Verification items for the finished model (mm, model axes). A direction names the side the tool comes from. Round coordinates to 2 decimals unless told otherwise and drop trailing zeros. Write each loop counter-clockwise with the first axis right and the second up, starting at its lowest first coordinate (ties: lowest second). Pieces come first, ordered by that corner, then holes. Notation, with made-up numbers: (45.5, 64) - (84.5, 64) arc R22 cw to (84.5, 89) - close; hole circle Ø11 at (25.5, -6.75). An arc over 180 degrees is marked (long way). Write each question's results on one line, items separated by ' | '.
```python
from build123d import *

# Parameters (mm, degrees)
SKETCH_1_W          = 96
SKETCH_1_H          = 45
SKETCH_1_R          = 1.75
EXTRUDE_1_DEPTH     = 4
SKETCH_2_W          = 4
SKETCH_2_H          = 45
EXTRUDE_2_DEPTH     = 85
SKETCH_3_W          = 49
SKETCH_3_H          = 45
EXTRUDE_3_DEPTH     = 4
SKETCH_4_W          = 41
SKETCH_4_H          = 4
EXTRUDE_4_DEPTH     = 45
FILLET_1_R          = 4
SKETCH_5_R          = 4.5
CUT_EXTRUDE_1_DEPTH = 4
FILLET_2_R          = 2


with BuildPart() as part:
    # 草图1 → 凸台-拉伸1 (new body)
    with BuildSketch(Plane.XY):
        Rectangle(SKETCH_1_W, SKETCH_1_H)
        with Locations((8.5, 0)):
            Circle(SKETCH_1_R, mode=Mode.SUBTRACT)
        with Locations((-36.5, 0)):
            Circle(SKETCH_1_R, mode=Mode.SUBTRACT)
    extrude(amount=EXTRUDE_1_DEPTH)

    # 草图2 → 凸台-拉伸2 (add)
    with BuildSketch(Plane(origin=(0, 0, 0), x_dir=(-1, 0, 0), z_dir=(0, 0, -1))):
        with Locations((-31, 0)):
            Rectangle(SKETCH_2_W, SKETCH_2_H)
        with Locations((14, 0)):
            Rectangle(SKETCH_2_W, SKETCH_2_H)
    extrude(amount=EXTRUDE_2_DEPTH)

    # 草图3 → 凸台-拉伸3 (add)
    with BuildSketch(Plane(origin=(0, 0, -85), x_dir=(-1, 0, 0), z_dir=(0, 0, -1))):
        with Locations((-8.5, 0)):
            Rectangle(SKETCH_3_W, SKETCH_3_H)
    extrude(amount=EXTRUDE_3_DEPTH)

    # 草图4 → 凸台-拉伸4 (add)
    with BuildSketch(Plane.XZ.offset(22.5)):
        with Locations((8.5, -42)):
            Rectangle(SKETCH_4_W, SKETCH_4_H)
    extrude(amount=-EXTRUDE_4_DEPTH)

    # 圆角1
    fillet_1_edges = [part.edges().sort_by_distance(p)[0] for p in [
        (-16, 0, 0),
        (33, 0, 0),
        (33, 0, -89),
        (-16, 0, -89),
    ]]
    fillet(fillet_1_edges, radius=FILLET_1_R)

    # 草图5 → 切除-拉伸1 (cut)
    with BuildSketch(Plane(origin=(0, 0, -89), x_dir=(-1, 0, 0), z_dir=(0, 0, -1))):
        with Locations((-8.5, 0)):
            Circle(SKETCH_5_R)
    extrude(amount=-CUT_EXTRUDE_1_DEPTH, mode=Mode.SUBTRACT)

    # 圆角2
    fillet_2_edges = [part.edges().sort_by_distance(p)[0] for p in [
        (-48, 0, 4),
        (-48, 0, 0),
        (48, 0, 4),
        (48, 0, 0),
    ]]
    fillet(fillet_2_edges, radius=FILLET_2_R - 0.0001)  # a hair under: the kernel refuses the full size


solid = part.part
```
(1) Go/stop test with flat-tipped pins: pin 1 Ø13.5 at (y, z) = (-9.5, -41.5) entering from -X; pin 2 Ø4 at (x, y) = (37, 2) entering from -Z; pin 3 Ø2 at (x, y) = (8.5, 0) entering from -Z. Record where each tip stops, or that it passes through.
Answer:
pin 1: x = -16 | pin 2: z = -0.54 | pin 3: z = -44
(2) Mould release check, pull along X, two halves, no side actions. Record for faces 5 (the cylindrical face through (4.208, 1.352, -87.028)), 6 (the flat face through (33, 0, -44)), 7 (the cylindrical face through (-14.797, 0.315, -87.859)): released by +X, released by -X, zero draft, split by the parting line, or undercut.
Answer:
face 5: undercut | face 6: released by +X | face 7: released by -X
(3) Thickness scan on L1, parallel to Z at x = -8.5, y = -5; L2, parallel to Y at x = 8, z = -86; L3, parallel to X at y = 3.5, z = -66. Record the ranges inside material, lowest first.
Answer:
L1: -89 to -85, -44 to -40, 0 to 4 | L2: -22.5 to -4.47, 4.47 to 22.5 | L3: -16 to -12, 29 to 33
(4) Section check B-B (x = -10). Record the cut outline in (y, z), plus the area to 3 significant figures.
Answer:
outline: (-22.5, -89) - (22.5, -89) - (22.5, -85) - (-22.5, -85) - close; (-22.5, -44) - (22.5, -44) - (22.5, -40) - (-22.5, -40) - close; (-22.5, 0) - (22.5, 0) - (22.5, 4) - (-22.5, 4) - close | area: 540 mm2
(5) Set-up check for faces 1 (the flat face through (41, 0, 0)), 2 (the cylindrical face through (10.169, 0.526, 1.972)), 3 (the flat face through (-12, 0, -20)), 4 (the flat face through (-33, 0, 0)): record each of +Z, -Z, +X, -X, +Y, -Y from which the full face is reachable in a straight line by a thin tool's end or side.
Answer:
face 1: -Z, +X, +Y, -Y | face 2: +Z | face 3: +Y, -Y | face 4: -Z, -X, +Y, -Y
(6) Section check A-A (x = 8.5). Record the cut outline in (y, z).
Answer:
outline: (-22.5, -89) - (-4.5, -89) - (-4.5, -85) - (-22.5, -85) - close; (-22.5, -44) - (22.5, -44) - (22.5, -40) - (-22.5, -40) - close; (-22.5, 0) - (-1.75, 0) - (-1.75, 4) - (-22.5, 4) - close; (1.75, 0) - (22.5, 0) - (22.5, 4) - (1.75, 4) - close; (4.5, -89) - (22.5, -89) - (22.5, -85) - (4.5, -85) - close
(7) Section check D-D (z = -28.5). Record the cut outline in (x, y), plus the area to 3 significant figures.
Answer:
outline: (-16, -22.5) - (-12, -22.5) - (-12, 22.5) - (-16, 22.5) - close; (29, -22.5) - (33, -22.5) - (33, 22.5) - (29, 22.5) - close | area: 360 mm2
(8) Section check C-C (y = 20). State how many separate pieces and enclosed holes the cut face has, plus the area to 3 significant figures.
Answer:
separate pieces: 1 | enclosed holes: 2 | area: 1,420 mm2
